Check sheet for the modelled part. Datum: model origin and axes. Units: mm. A direction names the side the tool comes from. Coordinates: 2 decimals unless noted, no trailing zeros. Loops run counter-clockwise (first coordinate to the right, second up) from the corner with the lowest first, then second, coordinate; pieces in that order, holes last. Notation, with made-up numbers: (45.5, -32.75) -> (93.5, -32.75) arc R11 cw to (93.5, -16.75) -> close; hole circle Ø3 at (-37, 65). An arc over 180 degrees is marked (long way). Use one line per item in the form item = value.
from build123d import *

# Parameters (mm, degrees)
SKETCH1_R           = 2.5
BOSS_EXTRUDE1_DEPTH = 5
SKETCH3_R           = 0.1
BOSS_EXTRUDE2_DEPTH = 0.1


with BuildPart() as part:
    # Sketch1 → Boss-Extrude1 (new body)
    with BuildSketch(Plane.XY):
        with BuildLine():
            Line((3.912222702, 3.113601376), (163.912222702, 3.113601376))
            ThreePointArc((163.912222702, 3.113601376), (172.824445404, 0), (163.912222702, -3.113601376))
            Line((163.912222702, -3.113601376), (3.912222702, -3.113601376))
            ThreePointArc((3.912222702, -3.113601376), (-5, 0), (3.912222702, 3.113601376))
        make_face()
        Circle(SKETCH1_R, mode=Mode.SUBTRACT)
    extrude(amount=BOSS_EXTRUDE1_DEPTH)

    # Sketch3 → Boss-Extrude2 (add)
    with BuildSketch(Plane(origin=(0, 0, 0), x_dir=(-1, 0, 0), z_dir=(0, 0, -1))):
        with Locations(Location((-167.824445404, 0, 0), (0, 0, 180))):
            Circle(SKETCH3_R)
    extrude(amount=BOSS_EXTRUDE2_DEPTH)


solid = part.part
(1) Section check A-A, the plane x = 0. Record the boundary of the cut face in (y, z), plus the area to 3 significant figures.
Established:
outline = (-5, 0) -> (-2.5, 0) -> (-2.5, 5) -> (-5, 5) -> close; (2.5, 0) -> (5, 0) -> (5, 5) -> (2.5, 5) -> close
area = 25.0 mm²
(2) Scan lines: line 1 along X through (y, z) = (-0.25, 1.5); line 2 along Y through (x, z) = (0, 1.9); line 3 along Z through (x, y) = (137.5, 2.75). Record each from-to range of solid material in increasing order.
Established:
line_1 = -4.99 to -2.49, 2.49 to 172.82
line_2 = -5 to -2.5, 2.5 to 5
line_3 = 0 to 5
(3) Go/stop test with flat-tipped pins: P1, Ø5, axis at x = 35, y = -3, coming from the -Z side; P2, Ø2, axis at x = 33.5, z = 4.5, coming from the +Y side; P3, Ø2.5, axis at x = 46.5, z = 1.5, coming from the -Y side. Record where each tip stops, or that it passes through.
Established:
P1 = 0
P2 = 3.11
P3 = -3.11
(4) Tool access check on faces 3 (the cylindrical face through (172.82, 0.17, 2.46)), 4 (the flat face through (85, -3.114, 2)). Record the directions out of +Z, -Z, +X, -X, +Y, -Y that give a thin tool (end or side, any length) a straight path to the whole face; none if there is none.
Established:
face_3 = +Z, -Z
face_4 = +Z, -Z, -Y
(5) Section check B-B, the plane z = 2.95. Record the boundary of the cut face in (x, y), plus the area to 3 significant figures.
Established:
outline = (3.91, -3.11) -> (163.91, -3.11) arc R5 ccw (long way) to (163.91, 3.11) -> (3.91, 3.11) arc R5 ccw (long way) to start; hole circle Ø5 at (0, 0)
area = 1,120 mm²
(6) Mould release check, pull along X, two halves, no side actions. Record for faces 1 (the flat face through (83, 3.114, 2)), 2 (the flat face through (85, 0, 5)): +X half, -X half, draft (parallel to the pull), parting line (faces both ways), or undercut.
Established:
face_1 = undercut
face_2 = draft
(7) Section check C-C, the plane x = 70.5. Record the boundary of the cut face in (y, z).
Established:
outline = (-3.11, 0) -> (3.11, 0) -> (3.11, 5) -> (-3.11, 5) -> close
